from build123d import *

# Parameters (mm, degrees)
F0_R     = 4.95
F0_R_2   = 4.2
F1_DEPTH = 5.4
F0_R_3   = 10.95
F0_R_4   = 1.25
F2_DEPTH = 3.7


# Not quite as in the source:
# - the program builds the solid bodies; features that only make, move or delete a surface that nothing else refers to are left out


with BuildPart() as f1:
    # F0 (on Front) → F1 (new body)
    with BuildSketch(Plane.XZ):
        Circle(F0_R)
        Circle(F0_R_2, mode=Mode.SUBTRACT)
    extrude(amount=F1_DEPTH)

    # F0 (on Front) → F2 (join)
    with BuildSketch(Plane.XZ):
        Circle(F0_R_3)
        with Locations((0, -8.2)):
            Circle(F0_R_4, mode=Mode.SUBTRACT)
        with Locations((-8.2, 0)):
            Circle(F0_R_4, mode=Mode.SUBTRACT)
        Circle(F0_R, mode=Mode.SUBTRACT)
        with Locations((8.2, 0)):
            Circle(F0_R_4, mode=Mode.SUBTRACT)
        with Locations((0, 8.2)):
            Circle(F0_R_4, mode=Mode.SUBTRACT)
    extrude(amount=F2_DEPTH)


solid = f1.part
The model under review builds one solid part; all positions refer to its coordinate system, in mm. A direction names the side the tool comes from. Round coordinates to 2 decimals unless told otherwise and drop trailing zeros. Write each loop counter-clockwise with the first axis right and the second up, starting at its lowest first coordinate (ties: lowest second). Pieces come first, ordered by that corner, then holes. Notation, with made-up numbers: M 78,-13 L 113,-13 A19 cw 113,7 Z; hole C 84.25,0.25 d11. An arc over 180 degrees is marked long. Use a Markdown table: item, result. Add a question column.
Q1. We need section D-D, the plane z = 3.75. State the section outline as (x, y) points.
Q2. We need section B-B, the plane x = 0. State the section outline as (y, z) points, plus the area to 3 significant figures.
Q3. We need section A-A, the plane z = 0. State the section outline as (x, y) points.
Q4. Machinability: for faces 5 (the face through (5, -3.7, -2)), 6 (the face through (0.672, -1.824, 9.254)), which of the approach directions +Z, -Z, +X, -X, +Y, -Y give a long, thin tool a straight path to every point of the face, cutting with its end or side? Answer none if there is none.
Q5. To check wall thickness, follow line 1 (Z direction, x = 0, y = -1.85); line 2 (X direction, y = -0.8, z = 1); line 3 (Z direction, x = -8.2, y = -0.75). State the ranges of each line that lie inside material, in increasing order.
Q6. We need section C-C, the plane y = -0.7. State the section outline as (x, z) points, plus the area to 3 significant figures.
Q7. The part is to be moulded in two halves that separate along X. For faces 1 (the face through (4.006, -2.662, 1.262)), 2 (the face through (5, 0, 0)), 3 (the face through (-9.121, -1.824, 0.845)), 4 (the face through (4.72, -4.54, 1.49)), say which applies: pulls with the +X half, pulls with the -X half, needs draft (parallel to the pull), parting line crosses it, or undercut.
Q8. Insertion check: pin 1 (4 mm diameter, centred on x = 8.2, z = 0, fed in from -Y); pin 2 (11 mm diameter, centred on x = 0, z = 0, fed in from -Y); pin 3 (3 mm diameter, centred on x = 8.5, y = -2, fed in from +Z); pin 4 (1.5 mm diameter, centred on y = -1.5, z = -7.5, fed in from +X). Each pin has a flat end and moves straight along its axis. Give the tip position at first contact, or say it passes through.
Findings below:
| question | item | result |
|---|---|---|
| 1 | outline | M -10.29,-3.7 L -3.23,-3.7 L -3.23,-5.4 L -1.89,-5.4 L -1.89,0 L -10.29,0 Z; M 1.89,-5.4 L 3.23,-5.4 L 3.23,-3.7 L 10.29,-3.7 L 10.29,0 L 1.89,0 Z |
| 2 | outline | M -5.4,-4.95 L -3.7,-4.95 L -3.7,-6.95 L 0,-6.95 L 0,-4.2 L -5.4,-4.2 Z; M -5.4,4.2 L 0,4.2 L 0,6.95 L -3.7,6.95 L -3.7,4.95 L -5.4,4.95 Z; M -3.7,-10.95 L 0,-10.95 L 0,-9.45 L -3.7,-9.45 Z; M -3.7,9.45 L 0,9.45 L 0,10.95 L -3.7,10.95 Z |
| 2 | area | 34.0 mm² |
| 3 | outline | M -10.95,-3.7 L -9.45,-3.7 L -9.45,0 L -10.95,0 Z; M -6.95,-3.7 L -4.95,-3.7 L -4.95,-5.4 L -4.2,-5.4 L -4.2,0 L -6.95,0 Z; M 4.2,-5.4 L 4.95,-5.4 L 4.95,-3.7 L 6.95,-3.7 L 6.95,0 L 4.2,0 Z; M 9.45,-3.7 L 10.95,-3.7 L 10.95,0 L 9.45,0 Z |
| 4 | face 5 | -Y |
| 4 | face 6 | +Y, -Y |
| 5 | line 1 | z = -10.95 to -9.45, -6.95 to -4.2, 4.2 to 6.95, 9.45 to 10.95 |
| 5 | line 2 | x = -10.9 to -8.95, -7.45 to -4.08, 4.08 to 7.45, 8.95 to 10.9 |
| 5 | line 3 | z = -7.26 to -1.25, 1.25 to 7.26 |
| 6 | outline | C 0,0 d21.9; hole C -8.2,0 d2.5; hole C 0,0 d8.4; hole C 0,-8.2 d2.5; hole C 0,8.2 d2.5; hole C 8.2,0 d2.5 |
| 6 | area | 302 mm² |
| 7 | face 1 | undercut |
| 7 | face 2 | needs draft |
| 7 | face 3 | undercut |
| 7 | face 4 | parting line crosses it |
| 8 | pin 1 | stops at y = -3.7 |
| 8 | pin 2 | stops at y = -5.4 |
| 8 | pin 3 | stops at z = 8.42 |
| 8 | pin 4 | stops at x = 8.62 |
